Can you work these out from the model? Positions are in its coordinate system, mm. A direction names the side the tool comes from. Round coordinates to 2 decimals unless told otherwise and drop trailing zeros. Loops run counter-clockwise (first coordinate to the right, second up) from the corner with the lowest first, then second, coordinate; pieces in that order, holes last. Notation, with made-up numbers: M 0.5,-3.5 L 56.5,-3.5 A19 ccw 56.5,11.5 Z; hole C 39,9.25 d7. An arc over 180 degrees is marked long. Answer as CSV lines item,"result".
from build123d import *

# Parameters (mm, degrees)
F0_W          = 46
F0_H          = 66
F0_W_2        = 36
F0_H_2        = 58
F1_DEPTH      = 3
F2_W          = 2
F2_H          = 61
F2_H_2        = 5
F3_DEPTH      = 11
F5_DEPTH      = 2
F6_W          = 12
F6_H          = 10
F7_DEPTH      = 5
F7_DEPTH_BACK = 5
F8_R          = 1.5
F9_DEPTH      = 10
F10_R         = 1
F11_DEPTH     = 11.8829661115
F12_DEPTH     = 10
F14_DEPTH     = 2
F16_DEPTH     = 2
F17_R         = 5
F18_SIZE      = 2


with BuildPart() as f1:
    # F0 (on Top) → F1 (new body)
    with BuildSketch(Plane.XY):
        Rectangle(F0_W, F0_H)
        with Locations((0, 1)):
            Rectangle(F0_W_2, F0_H_2, mode=Mode.SUBTRACT)
    extrude(amount=F1_DEPTH)

    # F2 (on face) → F3 (join)
    with BuildSketch(Plane(origin=(0, 0, 0), x_dir=(1, 0, 0), z_dir=(0, 0, -1))):
        with Locations((-22, -2.5)):
            Rectangle(F2_W, F2_H)
        Polygon((18, 28), (21, 28), (21, 33), (-23, 33), (-23, 28), (-21, 28), (-18, 28), align=None)
        with Locations((22, -2.5)):
            Rectangle(F2_W, F2_H)
        with Locations((22, 30.5)):
            Rectangle(F2_W, F2_H_2)
    extrude(amount=F3_DEPTH)

    # F4 (on face) → F5 (cut, through all)
    with BuildSketch(Plane.YZ.offset(23)):
        with BuildLine():
            Line((-26.4700967818, -11), (-7.943155244, -11))
            Line((-7.943155244, -11), (-7.943155244, -8.2140678056))
            ThreePointArc((-7.943155244, -8.2140678056), (-9.4076213381, -4.6785338996), (-12.943155244, -3.2140678056))
            Line((-12.943155244, -3.2140678056), (-21.4700967818, -3.2140678056))
            ThreePointArc((-21.4700967818, -3.2140678056), (-25.0056306878, -4.6785338996), (-26.4700967818, -8.2140678056))
            Line((-26.4700967818, -8.2140678056), (-26.4700967818, -11))
        make_face()
    extrude(amount=-F5_DEPTH, mode=Mode.SUBTRACT)

    # F6 (on face) → F7 (join, two sides)
    with BuildSketch(Plane.XZ.offset(33)) as f7_sk:
        with Locations((0, -2)):
            Rectangle(F6_W, F6_H)
        Polygon((23, -11), (6, -7), (-6, -7), (-23, -11), (-6, -16), (6, -16), align=None)
    extrude(amount=F7_DEPTH)
    extrude(f7_sk.sketch, amount=-F7_DEPTH_BACK)

    # F8 (on face) → F9 (cut, through all)
    with BuildSketch(Plane.XZ.offset(38)):
        with Locations((0, -10)):
            Circle(F8_R)
    extrude(amount=-F9_DEPTH, mode=Mode.SUBTRACT)

    # F10 (on face) → F11 (cut, through all)
    with BuildSketch(Plane.XY.offset(3)):
        with Locations((0, -33.5)):
            Circle(F10_R)
    extrude(amount=-F11_DEPTH, mode=Mode.SUBTRACT)

    # F12 (add): a face of the model
    f12_faces = [f1.faces().sort_by_distance(p)[0] for p in [
        (-22, 2.5, -11),
    ]]
    extrude(f12_faces, amount=F12_DEPTH)

    # F13 (on face) → F14 (cut, through all)
    with BuildSketch(Plane(origin=(-23, 0, 0), x_dir=(0, -1, 0), z_dir=(-1, 0, 0))):
        with BuildLine():
            ThreePointArc((-25.4259229114, -7), (-29.4259229114, -11), (-25.4259229114, -15))
            Line((-25.4259229114, -15), (-11.899846606, -15))
            ThreePointArc((-11.899846606, -15), (-7.899846606, -11), (-11.899846606, -7))
            Line((-11.899846606, -7), (-25.4259229114, -7))
        make_face()
    extrude(amount=-F14_DEPTH, mode=Mode.SUBTRACT)

    # F15 (on face) → F16 (join)
    with BuildSketch(Plane(origin=(-23, 0, 0), x_dir=(0, -1, 0), z_dir=(-1, 0, 0))):
        with BuildLine():
            ThreePointArc((-25.4259229114, -4), (-32.4259229114, -11), (-25.4259229114, -18))
            Line((-25.4259229114, -18), (-11.899846606, -18))
            ThreePointArc((-11.899846606, -18), (-4.899846606, -11), (-11.899846606, -4))
            Line((-11.899846606, -4), (-25.4259229114, -4))
        make_face()
        with BuildLine():
            Line((-11.899846606, -15), (-25.4259229114, -15))
            ThreePointArc((-25.4259229114, -15), (-29.4259229114, -11), (-25.4259229114, -7))
            Line((-25.4259229114, -7), (-11.899846606, -7))
            ThreePointArc((-11.899846606, -7), (-7.899846606, -11), (-11.899846606, -15))
        make_face(mode=Mode.SUBTRACT)
    extrude(amount=F16_DEPTH)

    # F17
    f17_edges = [f1.edges().sort_by_distance(p)[0] for p in [
        (-22, -28, -21),
    ]]
    fillet(f17_edges, radius=F17_R)

    # F18
    f18_edges = [f1.edges().sort_by_distance(p)[0] for p in [
        (6, -35.5, 3),
        (-6, -35.5, 3),
    ]]
    chamfer(f18_edges, length=F18_SIZE)


solid = f1.part
Item 1: If we section it at B-B on z = -2.25: Write out the boundary of the cut face in (x, y).
Output:
outline,"M -23,-33 L -6,-33 L -6,-38 L 6,-38 L 6,-33 L 23,-33 L 23,33 L 21,33 L 21,-28 L -21,-28 L -21,33 L -23,33 Z; hole C 0,-33.5 d2"
Item 2: If we section it at D-D on z = -12.5: Write out the boundary of the cut face in (x, y).
Output:
outline,"M -25,5.06 L -23,5.06 L -23,-28 L -21,-28 L -21,8.19 L -25,8.19 Z; M -25,29.13 L -21,29.13 L -21,33 L -23,33 L -23,32.26 L -25,32.26 Z; M -17.9,-38 L 17.9,-38 L 17.9,-28 L -17.9,-28 Z"
Item 3: If we section it at A-A on x = 0: Write out the boundary of the cut face in (y, z), then the cut area to 3 significant figures.
Output:
outline,"M -38,-16 L -28,-16 L -28,-11.5 L -38,-11.5 Z; M -38,-8.5 L -34.5,-8.5 L -34.5,3 L -38,3 Z; M -32.5,-8.5 L -28,-8.5 L -28,3 L -32.5,3 Z; M 30,0 L 33,0 L 33,3 L 30,3 Z"
area,"146 mm2"
Item 4: On a 3-axis mill with a long thin cutter (end or side, diameter ignored), from which of +Z, -Z, +X, -X, +Y, -Y can I reach the whole of each face in a straight line? I mean faces 1 (the face through (-22, -28, -13)), 2 (the face through (-23.99, 4.9, -11.15)), 3 (the face through (-23, 19, -7)), 4 (the face through (22, -7.943, -10)), 5 (the face through (-6, -35, -3)). Say none if no direction works.
Output:
face 1,"-Z, -X, -Y"
face 2,"-X, -Y"
face 3,"-X"
face 4,"-Z, +X"
face 5,"+Z, -X, -Y"
Item 5: If I drill on line 1 along X through (y, z) = (-12, 1.5); line 2 along X through (y, z) = (-33.5, -3); line 3 along Y through (x, z) = (0, -4.75), over which ranges is the centre line in solid material (lowest first)? Write a range as from..to.
Output:
line 1,"x = -23..-18, 18..23"
line 2,"x = -6..-1, 1..6"
line 3,"y = -38..-34.5, -32.5..-28"
Item 6: If we section it at C-C on y = -1.5: Write out the boundary of the cut face in (x, z).
Output:
outline,"M -23,-21 L -21,-21 L -21,0 L -18,0 L -18,3 L -23,3 Z; M 18,0 L 21,0 L 21,-11 L 23,-11 L 23,3 L 18,3 Z"
Item 7: Will these pins go through, and if not, where does the flat tip stop? pin 1 (2 mm diameter, centred on y = 8, z = -14, fed in from +X); pin 2 (5 mm diameter, centred on x = -1, y = -30.5, fed in from -Z); pin 3 (0.6 mm diameter, centred on x = -24, y = 19.5, fed in from -Z).
Output:
pin 1,"stops at x = -21"
pin 2,"stops at z = -16"
pin 3,"stops at z = -18"
Item 8: We'd pull the mould along Z, two halves only. Please class faces 6 (the face through (22, -27, -11)), 7 (the face through (5, -35, 2)), 8 (the face through (-0.325, -33.07, -11.464)), 9 (the face through (18, 1, 1)): released by +Z, released by -Z, zero draft, split by the parting line, or undercut.
Output:
face 6,"released by -Z"
face 7,"released by +Z"
face 8,"undercut"
face 9,"zero draft"
